Autodesk Inventor part; units mm, degrees
ref_plane "YZ Plane" through (0, 0, 0) normal (1, 0, 0) x (0, 1, 0)
ref_plane "XZ Plane" through (0, 0, 0) normal (0, 1, 0) x (-1, 0, 0)
ref_plane "XY Plane" through (0, 0, 0) normal (0, 0, 1) x (1, 0, 0)
sketch "スケッチ1" plane through (0, 0, 0) normal (0, 0, 1) x (1, 0, 0)
  line L0 (0, 0) -> (30, 0)
  line L1 (30, 0) -> (30, -1.6)
  line L2 (30, -1.6) -> (0, -1.6)
  arc A0 (-3.7104, 1.1971) -> (-1.0982, -1.2457) centre (-5, -2.8) ccw
  line L3 (0, 0) -> (-3.7104, 1.1971)
  line L4 (0, -1.6) -> (-1.0982, -1.2457)
  line L5 (0, 0) -> (0, -1.6) construction
  circle A1 centre (-5, -2.8) radius 1.5
  dimension "d0" = 1.6
  dimension "d1" = 30
  dimension "d2" = 8.4
  dimension "d4" = 35
  dimension "d5" = 2.8
  dimension "d6" = 3
extrude "押し出し1" add sketch "スケッチ1" along normal blind 100
sketch "スケッチ2" plane through (0, -1.6, 0) normal (0, -1, 0) x (1, 0, 0)
  line L0 (0, 100) -> (-3.7104, 100)
  line L1 (0, 100) -> (-10, 100)
  line L2 (-10, -0.2) -> (0, -0.2)
  line L3 (-10, 84) -> (0, 84)
  line L4 (0, 0) -> (0, 100)
  line L5 (-10, 39.8) -> (0, 39.8)
  line L6 (-10, 15.8) -> (0, 15.8)
  line L7 (16.4, 101.8084) -> (16.4, 1.6084) construction
  line L8 (30, 0) -> (30, 100) construction
  line L9 (30, 89) -> (16.4, 89) construction
  line L10 (30, 63) -> (16.4, 63) construction
  line L11 (30, 37) -> (16.4, 37) construction
  line L12 (30, 11) -> (16.4, 11) construction
  line L13 (30, 100) -> (0, 100) construction
  line L14 (22.3, 100) -> (22.3, 0) construction
  circle A0 centre (22.3, 89) radius 3.1
  circle A1 centre (16.4, 63) radius 3.1
  circle A2 centre (22.3, 37) radius 3.1
  circle A3 centre (16.4, 11) radius 3.1
  line L15 (30, 0) -> (0, 0) construction
  line L16 (-10, 60) -> (0, 60)
  line L17 (-10, 100) -> (-10, 84)
  line L18 (0, 84) -> (0, 100)
  line L19 (-10, 60) -> (-10, 39.8)
  line L20 (-10, 15.8) -> (-10, -0.2)
  line L21 (0, -0.2) -> (0, 15.8)
  line L22 (0, 39.8) -> (0, 60)
  dimension "d9" = 100.2
  dimension "d10" = 10
  dimension "d11" = 16
  dimension "d12" = 16
  dimension "d13" = 24
  dimension "d15" = 7.7
  dimension "d16" = 6.2
  dimension "d17" = 11
  dimension "d19" = 11
  dimension "d20" = 13.6
  dimension "d21" = 37
  dimension "d22" = 37
  dimension "d23" = 24
extrude "押し出し2" cut sketch "スケッチ2" along normal mid plane 100.2
properties part number "蝶番1"
Could you check a few things on this model? Use its own coordinates, in mm. A direction names the side the tool comes from. Coordinates: 2 decimals unless noted, no trailing zeros. Order: outer loops, then holes, each group sorted by start corner. A loop starts at its lowest first (then second) coordinate and runs counter-clockwise, first axis right, second up. Notation, with made-up numbers: (2, -9.75) - (48, -9.75) arc R33 cw to (48, 22.25) - close; hole circle Ø6 at (39, 4.25). An arc over 180 degrees is marked (long way). Answer in a Markdown table with one row per item. Add a question column.
(1) Will these pins go through, and if not, where does the flat tip stop? pin 1 (4 mm diameter, centred on x = -5, y = -2.8, fed in from -Z); pin 2 (0.5 mm diameter, centred on y = -0.5, z = 96, fed in from -X); pin 3 (8 mm diameter, centred on x = 16.4, z = 11, fed in from +Y).
(2) If we mould it in two halves opening along Y, with no side actions, what happens to faces 4 (the face through (15, -1.6, 49)), 5 (the face through (21.896, -0.811, 40.074)), 6 (the face through (-6.2, -1.9, 27.6))? For each: released by +Y, released by -Y, zero draft, split by the parting line, or undercut.
(3) I need wall thicknesses on L1, parallel to Z at x = 16.4, y = -0.8; L2, parallel to Z at x = -6.5, y = -0.25; L3, parallel to Y at x = -5, z = 71.25. Which ranges of each line are inside material? Lowest first, please.
(4) If we section it at A-A, the plane x = 22.3: Please give me the cut outline in (y, z).
(5) If we section it at C-C, the plane z = 80: Please give me the cut outline in (x, y), then the cut area to 3 significant figures.
(6) If we section it at D-D, the plane x = -5: Please give me the cut outline in (y, z).
(7) If we section it at B-B, the plane z = 37: Please give me the cut outline in (x, y), then the cut area to 3 significant figures.
(8) On a 3-axis mill with a long thin cutter (end or side, diameter ignored), from which of +Z, -Z, +X, -X, +Y, -Y can I reach the whole of each face in a straight line? I mean faces 1 (the face through (-3.6, -1.8, 39.8)), 2 (the face through (15, 0, 49)), 3 (the face through (-3.6, -1.8, 84)). Say none if no direction works.
Results are:
| question | item | result |
|---|---|---|
| 1 | pin 1 | stops at z = 15.8 |
| 1 | pin 2 | stops at x = 0 |
| 1 | pin 3 | stops at y = 0 |
| 2 | face 4 | released by -Y |
| 2 | face 5 | zero draft |
| 2 | face 6 | undercut |
| 3 | L1 | z = 0 to 7.9, 14.1 to 59.9, 66.1 to 100 |
| 3 | L2 | z = 15.8 to 39.8, 60 to 84 |
| 3 | L3 | y = -7 to -4.3, -1.3 to 1.4 |
| 4 | outline | (-1.6, 0) - (0, 0) - (0, 33.9) - (-1.6, 33.9) - close; (-1.6, 40.1) - (0, 40.1) - (0, 85.9) - (-1.6, 85.9) - close; (-1.6, 92.1) - (0, 92.1) - (0, 100) - (-1.6, 100) - close |
| 5 | outline | (-3.71, 1.2) arc R4.2 ccw (long way) to (-1.1, -1.25) - (0, -1.6) - (30, -1.6) - (30, 0) - (0, 0) - close; hole circle Ø3 at (-5, -2.8) |
| 5 | area | 99.2 mm2 |
| 6 | outline | (-7, 15.8) - (-4.3, 15.8) - (-4.3, 39.8) - (-7, 39.8) - close; (-7, 60) - (-4.3, 60) - (-4.3, 84) - (-7, 84) - close; (-1.3, 15.8) - (1.4, 15.8) - (1.4, 39.8) - (-1.3, 39.8) - close; (-1.3, 60) - (1.4, 60) - (1.4, 84) - (-1.3, 84) - close |
| 7 | outline | (-3.71, 1.2) arc R4.2 ccw (long way) to (-1.1, -1.25) - (0, -1.6) - (19.2, -1.6) - (19.2, 0) - (0, 0) - close; (25.4, -1.6) - (30, -1.6) - (30, 0) - (25.4, 0) - close; hole circle Ø3 at (-5, -2.8) |
| 7 | area | 89.3 mm2 |
| 8 | face 1 | -X, +Y, -Y |
| 8 | face 2 | +Z, -Z, +X, +Y |
| 8 | face 3 | +Z, -X, +Y, -Y |
